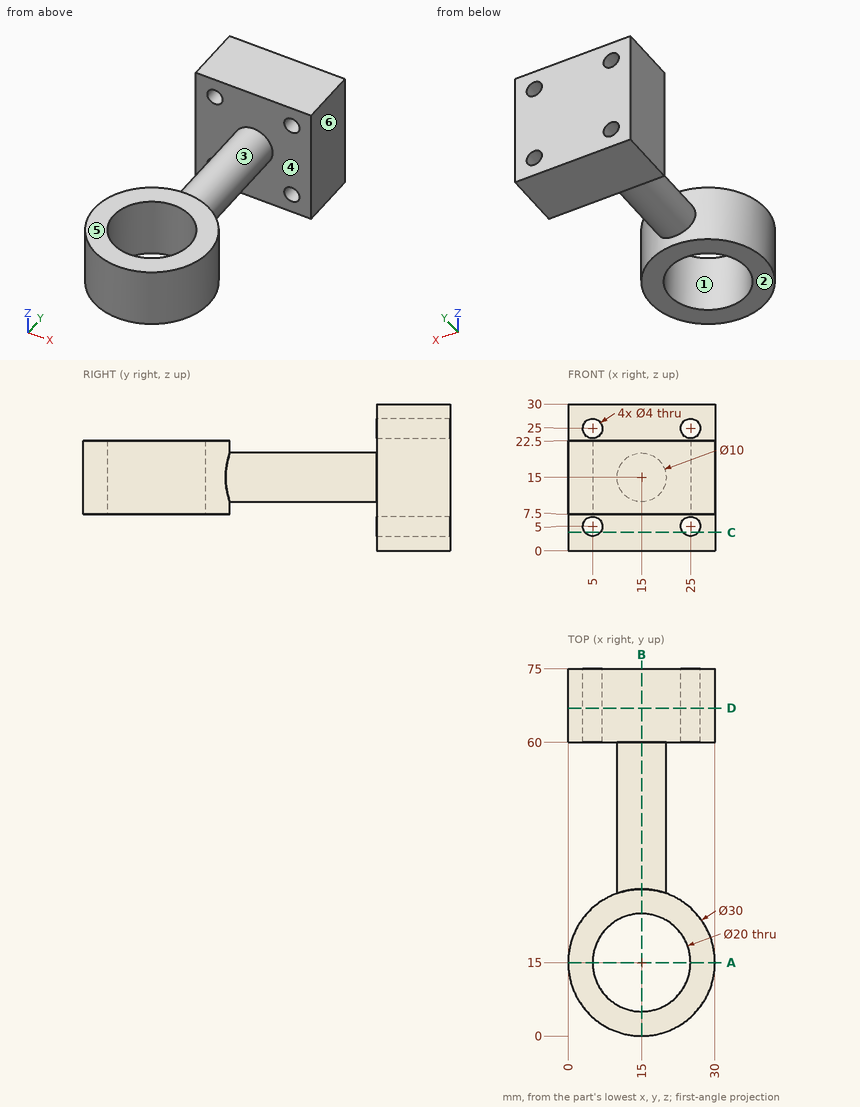
Geometry: see drawing. Coordinates: mm, zero at the bounding-box minimum. A direction names the side the tool comes from. Give positions to 0.01 mm unless a question says otherwise; leave off trailing zeros. Loops run counter-clockwise (first coordinate to the right, second up) from the corner with the lowest first, then second, coordinate; pieces in that order, holes last. Notation, with made-up numbers: (-8, 28.5) - (30, 28.5) arc R9 ccw to (30, 37.5) - close; hole circle Ø4 at (21.25, 28). An arc over 180 degrees is marked (long way). Use CSV: the item, a comma, the result in double quotes. Start each with the question number.
1. Section B-B (x = 15). Output: boundary loops of the cut face in (y, z).
2. Section D-D (y = 67). Output: boundary loops of the cut face in (x, z), then the cut area to 3 significant figures.
3. Section C-C (z = 3.75). Output: boundary loops of the cut face in (x, y).
4. Ray query, L1, parallel to X at y = 68, z = 5; L2, parallel to X at y = 41, z = 15.25; L3, parallel to Y at x = 26, z = 2. Return the intervals inside material, ascending.
5. Draft query along X for the marked faces 1, 2 and 3. Return one class per face: +X half, -X half, draft (parallel to the pull), parting line (faces both ways), or undercut.
6. Pin query (flat end, axial travel): pin 1 (1 mm diameter, centred on y = 9.5, z = 9.5, fed in from +X); pin 2 (10 mm diameter, centred on x = 5, z = 5.5, fed in from -Y); pin 3 (6 mm diameter, centred on x = 12, y = 32, fed in from -Z). Return the tip coordinate at first contact, or that it passes through.
7. Reachability of the marked faces 4, 5 and 6 from +Z, -Z, +X, -X, +Y, -Y: full face, straight path, thin tool, end or side. Return the list, or none.
8. Section A-A (y = 15). Output: boundary loops of the cut face in (x, z), then the cut area to 3 significant figures.
Response:
1,outline,"(0, 7.5) - (5, 7.5) - (5, 22.5) - (0, 22.5) - close; (25, 7.5) - (30, 7.5) - (30, 10) - (60, 10) - (60, 0) - (75, 0) - (75, 30) - (60, 30) - (60, 20) - (30, 20) - (30, 22.5) - (25, 22.5) - close"
2,outline,"(0, 0) - (30, 0) - (30, 30) - (0, 30) - close; hole circle Ø4 at (5, 5); hole circle Ø4 at (5, 25); hole circle Ø4 at (25, 5); hole circle Ø4 at (25, 25)"
2,area,"850 mm²"
3,outline,"(0, 60) - (3.44, 60) - (3.44, 75) - (0, 75) - close; (6.56, 60) - (23.44, 60) - (23.44, 75) - (6.56, 75) - close; (26.56, 60) - (30, 60) - (30, 75) - (26.56, 75) - close"
4,L1,"0 to 3, 7 to 23, 27 to 30"
4,L2,"10.01 to 19.99"
4,L3,"60 to 75"
5,face 1,"undercut"
5,face 2,"draft"
5,face 3,"parting line"
6,pin 1,"x = 29.14"
6,pin 2,"y = 1.01"
6,pin 3,"z = 7.5"
7,face 4,"none"
7,face 5,"+Z, +X, -X, -Y"
7,face 6,"+Z, -Z, +X, +Y, -Y"
8,outline,"(0, 7.5) - (5, 7.5) - (5, 22.5) - (0, 22.5) - close; (25, 7.5) - (30, 7.5) - (30, 22.5) - (25, 22.5) - close"
8,area,"150 mm²"
